Autodesk Inventor part; units mm, degrees
ref_plane "Work Plane1" through (0, 0, 0) normal (0, 0, 1) x (1, 0, 0)
ref_plane "Work Plane3" through (28, 0, 7.5) normal (1, 0, 0) x (0, 0, -1)
ref_plane "YZ Plane" through (0, 0, 0) normal (1, 0, 0) x (0, 1, 0)
sketch "Sketch1" plane through (0, 0, 0) normal (0, 0, 1) x (1, 0, 0)
  line L0 (0, 0) -> (56, 0)
  line L1 (56, 0) -> (56, 25)
  line L2 (56, 25) -> (0, 25)
  line L3 (0, 25) -> (0, 0)
  dimension "d0" = 56
  dimension "d1" = 25
extrude "Extrusion1" add sketch "Sketch1" along normal mid plane 15
sketch "Sketch2" plane through (0, 0, 7.5) normal (0, 0, 1) x (1, 0, 0)
  line L0 (0, 0) -> (56, 0)
  line L1 (0, 25) -> (0, 0)
  point P0 (15, 11)
  dimension "d4" = 11
  dimension "d5" = 15
hole "Hole1" at (15, 11, 7.5) direction (0, 0, -1) diameter 7 depth 15 counterbore diameter 8.5 counterbore depth 1
ref_plane "Work Plane1" through (0, 0, 0) normal (0, 0, 1) x (1, 0, 0)
sketch "Sketch3" plane through (0, 0, 0) normal (0, 0, 1) x (1, 0, 0)
  line L0 (1.4815, 11) -> (-8, 11)
  line L1 (-8, 11) -> (-8, 15)
  line L2 (-8, 15) -> (0, 15)
  line L3 (0, 16) -> (3, 16)
  line L4 (3, 16) -> (3, 11)
  line L5 (3, 11) -> (1.4815, 11)
  line L6 (0, 15) -> (0, 16)
  line L7 (0, 0) -> (0, 25)
  line L8 (56, 0) -> (0, 0)
  dimension "d14" = 8
  dimension "d15" = 11
  dimension "d16" = 3
  dimension "d17" = 11
  dimension "d18" = 10
revolve "Revolution1" add sketch "Sketch3" angle 360 about axis through (1.4815, 11, 0) along (-1, 0, 0)
sketch "Sketch4" plane through (-8, 11, 0) normal (-1, 0, 0) x (0, 0, 1)
  circle A0 centre (0, 0) radius 4
  point P0 (0, -11)
hole "Hole2" at (-8, 11, 0) direction (1, 0, 0) diameter 5 depth 11
thread "Thread1"
sketch "Sketch6" plane through (0, 0, 7.5) normal (0, -1, 0) x (1, 0, 0)
  line L0 (0, -15) -> (0, 0)
  line L1 (56, 0) -> (56, -15)
  line L2 (0, 0) -> (56, 0)
  point P0 (0, -7.5)
  point P1 (9, -7.5)
  point P2 (47, -7.5)
  point P3 (0, -7.5)
  point P4 (56, -7.5)
  point P5 (28, 0)
  dimension "d29" = 38
  dimension "d30" = 19
hole "Hole3" at (9, 0, 0) at (47, 0, 0) direction (0, 1, 0) diameter 3.242 depth 5
ref_plane "Work Plane3" through (28, 0, 7.5) normal (1, 0, 0) x (0, 0, -1)
sketch "Sketch8" plane through (28, 0, 7.5) normal (1, 0, 0) x (0, 0, -1)
  line L0 (15, 25) -> (0, 25)
  line L1 (15, 0) -> (15, 25)
  line L2 (9.8, 25) -> (4, 0)
  line L3 (0, 25) -> (0, 0)
  line L4 (15, 0) -> (0, 0)
  point P0 (7.5, 0)
  dimension "d40" = 5.2
  dimension "d41" = 4
sketch "Sketch10" plane through (0, 25, 7.5) normal (0, 1, 0) x (1, 0, 0)
  circle A0 centre (28, 9.8) radius 1.5
  point P0 (0, 7.5)
  dimension "d42" = 3
sweep "Sweep1" cut profiles "Sketch10" path "Sketch8" path curves L2
sketch "Sketch12" plane through (3, 11, 0) normal (-1, 0, 0) x (0, 0, 1)
  line L0 (-7.5, 14) -> (7.5, 14)
  line L1 (7.5, -11) -> (7.5, 14)
  line L2 (7.5, -11) -> (-7.5, -11)
  line L3 (-7.5, 14) -> (-7.5, -11)
  circle A0 centre (0, 0) radius 1.5
  point P0 (0, -11)
  point P1 (0, 14)
  dimension "d45" = 3
  dimension "d46" = 11
extrude "Extrusion2" cut sketch "Sketch12" against normal blind 32 contours A0
properties part number "150" material "Steel, Cast"
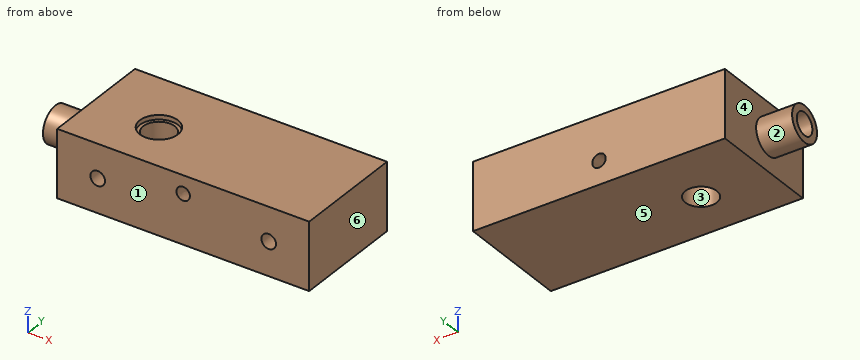
Part model, mm, in its own coordinate system. Face numbers are marked on the shaded views. A direction names the side the tool comes from. Round coordinates to 2 decimals unless told otherwise and drop trailing zeros. Loops run counter-clockwise (first coordinate to the right, second up) from the corner with the lowest first, then second, coordinate; pieces in that order, holes last. Notation, with made-up numbers: (77.25, 12.5) -> (97.25, 12.5) arc R23 ccw to (97.25, 22.5) -> close; hole circle Ø10 at (43.25, -39). An arc over 180 degrees is marked (long way). Use a Markdown table: item, result.
1) Cut at B-B, the plane x = 47. List the corners of the cut face in (y, z).
The answers:
| item | result |
|---|---|
| outline | (0, -7.5) -> (25, -7.5) -> (25, 7.5) -> (0, 7.5) -> (0, 1.62) -> (5, 1.62) -> (5, -1.62) -> (0, -1.62) -> close |
2) Pull direction X, two halves, no side cores. Call the marked faces 3, 4, 5 and 6: pulls with the +X half, pulls with the -X half, needs draft (parallel to the pull), parting line crosses it, or undercut.
The answers:
| item | result |
|---|---|
| face 3 | undercut |
| face 4 | pulls with the -X half |
| face 5 | needs draft |
| face 6 | pulls with the +X half |
3) Cut at D-D, the plane x = 16. List the corners of the cut face in (y, z).
The answers:
| item | result |
|---|---|
| outline | (0, -7.5) -> (7.65, -7.5) -> (7.65, 6.5) -> (6.87, 6.5) -> (6.87, 7.5) -> (0, 7.5) -> close; (14.35, -7.5) -> (25, -7.5) -> (25, 7.5) -> (15.13, 7.5) -> (15.13, 6.5) -> (14.35, 6.5) -> close |
4) Tool access for the marked faces 1 and 2: list every direction of +Z, -Z, +X, -X, +Y, -Y with a clear straight run to the whole face (end or side of a thin tool).
The answers:
| item | result |
|---|---|
| face 1 | +Z, -Z, +X, -X, -Y |
| face 2 | -X |
5) Cut at C-C, the plane y = 11. State how many separate pieces and enclosed holes the cut face has, and give its area (3 significant figures).
The answers:
| item | result |
|---|---|
| separate pieces | 3 |
| enclosed holes | 0 |
| area | 666 mm2 |
6) Cut at A-A, the plane x = 9. List the corners of the cut face in (y, z), and give its area (3 significant figures).
The answers:
| item | result |
|---|---|
| outline | (0, -7.5) -> (25, -7.5) -> (25, 7.5) -> (0, 7.5) -> (0, 1.62) -> (5, 1.62) -> (5, -1.62) -> (0, -1.62) -> close; hole circle Ø3 at (11, 0) |
| area | 352 mm2 |
7) Probe line 1 (X direction, y = 2.9, z = 0); line 2 (Y direction, x = 15, z = 6.8); line 3 (Y direction, x = 0.5, z = 0). List the from-to ranges inside material, lowest first. Write a range as [from, to].
The answers:
| item | result |
|---|---|
| line 1 | x = [0, 7.38], [10.62, 45.38], [48.62, 56] |
| line 2 | y = [0, 6.75], [15.25, 25] |
| line 3 | y = [0, 8.5], [13.5, 25] |
8) Drop flat-ended pins along their axis: pin 1 Ø5.5 at (y, z) = (10.5, 0.5) entering from -X; pin 2 Ø3.5 at (y, z) = (11, 0) entering from -X; pin 3 Ø8 at (y, z) = (17.5, -5.5) entering from -X; pin 4 Ø2.5 at (y, z) = (11, 0) entering from -X. Give the stop position or say it passes through.
The answers:
| item | result |
|---|---|
| pin 1 | stops at x = -8 |
| pin 2 | stops at x = 3 |
| pin 3 | stops at x = 0 |
| pin 4 | stops at x = 35 |
